For this review, take the finished solid that the model builds, in its own axes (mm). Round coordinates to 2 decimals unless told otherwise and drop trailing zeros.
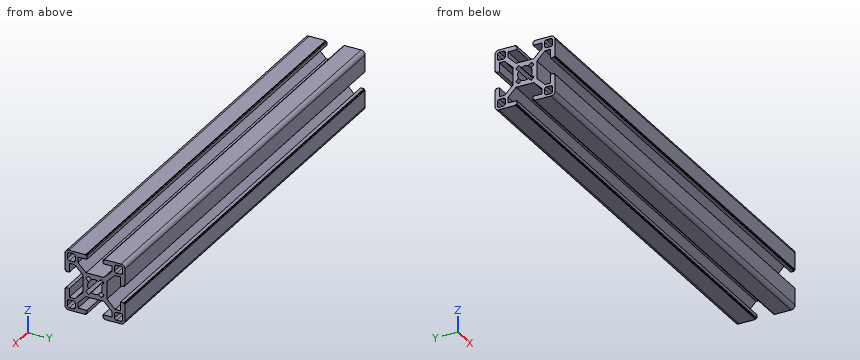
from build123d import *

# Parameters (mm, degrees)
AUFSATZ_LINEAR_AUSTRAGEN1_DEPTH = 220


with BuildPart() as part:
    # Skizze1 → Aufsatz-Linear austragen1 (new body)
    with BuildSketch(Plane(origin=(0, 0, 0), x_dir=(0, 0, -1), z_dir=(1, 0, 0))):
        with BuildLine():
            Line((10.055634919, 8.5), (12.8, 8.5))
            Line((12.8, 8.5), (12.8, 4.05))
            Line((12.8, 4.05), (14.5, 4.05))
            Line((14.5, 4.05), (14.5, 4.651637069))
            Line((14.5, 4.651637069), (15, 4.651637069))
            Line((15, 4.651637069), (15, 13))
            ThreePointArc((15, 13), (14.414213562, 14.414213562), (13, 15))
            Line((13, 15), (4.651637069, 15))
            Line((4.651637069, 15), (4.651637069, 14.5))
            Line((4.651637069, 14.5), (4.05, 14.5))
            Line((4.05, 14.5), (4.05, 12.8))
            Line((4.05, 12.8), (8.5, 12.8))
            Line((8.5, 12.8), (8.5, 10.055634919))
            Line((8.5, 10.055634919), (4.444365081, 6))
            Line((4.444365081, 6), (-4.444365081, 6))
            Line((-4.444365081, 6), (-8.5, 10.055634919))
            Line((-8.5, 10.055634919), (-8.5, 12.8))
            Line((-8.5, 12.8), (-4.05, 12.8))
            Line((-4.05, 12.8), (-4.05, 14.5))
            Line((-4.05, 14.5), (-4.651637069, 14.5))
            Line((-4.651637069, 14.5), (-4.651637069, 15))
            Line((-4.651637069, 15), (-13, 15))
            ThreePointArc((-13, 15), (-14.414213562, 14.414213562), (-15, 13))
            Line((-15, 13), (-15, 4.651637069))
            Line((-15, 4.651637069), (-14.5, 4.651637069))
            Line((-14.5, 4.651637069), (-14.5, 4.05))
            Line((-14.5, 4.05), (-12.8, 4.05))
            Line((-12.8, 4.05), (-12.8, 8.5))
            Line((-12.8, 8.5), (-10.055634919, 8.5))
            Line((-10.055634919, 8.5), (-6, 4.444365081))
            Line((-6, 4.444365081), (-6, -4.444365081))
            Line((-6, -4.444365081), (-10.055634919, -8.5))
            Line((-10.055634919, -8.5), (-12.8, -8.5))
            Line((-12.8, -8.5), (-12.8, -4.05))
            Line((-12.8, -4.05), (-14.5, -4.05))
            Line((-14.5, -4.05), (-14.5, -4.651637069))
            Line((-14.5, -4.651637069), (-15, -4.651637069))
            Line((-15, -4.651637069), (-15, -13))
            ThreePointArc((-15, -13), (-14.414213562, -14.414213562), (-13, -15))
            Line((-13, -15), (-4.651637069, -15))
            Line((-4.651637069, -15), (-4.651637069, -14.5))
            Line((-4.651637069, -14.5), (-4.05, -14.5))
            Line((-4.05, -14.5), (-4.05, -12.8))
            Line((-4.05, -12.8), (-8.5, -12.8))
            Line((-8.5, -12.8), (-8.5, -10.055634919))
            Line((-8.5, -10.055634919), (-4.444365081, -6))
            Line((-4.444365081, -6), (4.444365081, -6))
            Line((4.444365081, -6), (8.5, -10.055634919))
            Line((8.5, -10.055634919), (8.5, -12.8))
            Line((8.5, -12.8), (4.05, -12.8))
            Line((4.05, -12.8), (4.05, -14.5))
            Line((4.05, -14.5), (4.651637069, -14.5))
            Line((4.651637069, -14.5), (4.651637069, -15))
            Line((4.651637069, -15), (13, -15))
            ThreePointArc((13, -15), (14.414213562, -14.414213562), (15, -13))
            Line((15, -13), (15, -4.651637069))
            Line((15, -4.651637069), (14.5, -4.651637069))
            Line((14.5, -4.651637069), (14.5, -4.05))
            Line((14.5, -4.05), (12.8, -4.05))
            Line((12.8, -4.05), (12.8, -8.5))
            Line((12.8, -8.5), (10.055634919, -8.5))
            Line((10.055634919, -8.5), (6, -4.444365081))
            Line((6, -4.444365081), (6, 4.444365081))
            Line((6, 4.444365081), (10.055634919, 8.5))
        make_face()
        with BuildLine():
            ThreePointArc((12.8, 13.8), (13.507106781, 13.507106781), (13.8, 12.8))
            Line((13.8, 12.8), (13.8, 10.8))
            ThreePointArc((13.8, 10.8), (13.507106781, 10.092893219), (12.8, 9.8))
            Line((12.8, 9.8), (10.8, 9.8))
            ThreePointArc((10.8, 9.8), (10.092893219, 10.092893219), (9.8, 10.8))
            Line((9.8, 10.8), (9.8, 12.8))
            ThreePointArc((9.8, 12.8), (10.092893219, 13.507106781), (10.8, 13.8))
            Line((10.8, 13.8), (12.8, 13.8))
        make_face(mode=Mode.SUBTRACT)
        with BuildLine():
            Line((-3.117157854, 4.531371416), (-1.775079755, 3.189293317))
            ThreePointArc((-1.775079755, 3.189293317), (0, 3.65), (1.775079755, 3.189293317))
            Line((1.775079755, 3.189293317), (3.117157854, 4.531371416))
            ThreePointArc((3.117157854, 4.531371416), (3.889087297, 3.889087297), (4.531371416, 3.117157854))
            Line((4.531371416, 3.117157854), (3.189293317, 1.775079755))
            ThreePointArc((3.189293317, 1.775079755), (3.65, 0), (3.189293317, -1.775079755))
            Line((3.189293317, -1.775079755), (4.531371416, -3.117157854))
            ThreePointArc((4.531371416, -3.117157854), (3.889087297, -3.889087297), (3.117157854, -4.531371416))
            Line((3.117157854, -4.531371416), (1.775079755, -3.189293317))
            ThreePointArc((1.775079755, -3.189293317), (0, -3.65), (-1.775079755, -3.189293317))
            Line((-1.775079755, -3.189293317), (-3.117157854, -4.531371416))
            ThreePointArc((-3.117157854, -4.531371416), (-3.889087297, -3.889087297), (-4.531371416, -3.117157854))
            Line((-4.531371416, -3.117157854), (-3.189293317, -1.775079755))
            ThreePointArc((-3.189293317, -1.775079755), (-3.65, 0), (-3.189293317, 1.775079755))
            Line((-3.189293317, 1.775079755), (-4.531371416, 3.117157854))
            ThreePointArc((-4.531371416, 3.117157854), (-3.889087297, 3.889087297), (-3.117157854, 4.531371416))
        make_face(mode=Mode.SUBTRACT)
        with BuildLine():
            ThreePointArc((-13.8, 12.8), (-13.507106781, 13.507106781), (-12.8, 13.8))
            Line((-12.8, 13.8), (-10.8, 13.8))
            ThreePointArc((-10.8, 13.8), (-10.092893219, 13.507106781), (-9.8, 12.8))
            Line((-9.8, 12.8), (-9.8, 10.8))
            ThreePointArc((-9.8, 10.8), (-10.092893219, 10.092893219), (-10.8, 9.8))
            Line((-10.8, 9.8), (-12.8, 9.8))
            ThreePointArc((-12.8, 9.8), (-13.507106781, 10.092893219), (-13.8, 10.8))
            Line((-13.8, 10.8), (-13.8, 12.8))
        make_face(mode=Mode.SUBTRACT)
        with BuildLine():
            ThreePointArc((9.8, -10.8), (10.092893219, -10.092893219), (10.8, -9.8))
            Line((10.8, -9.8), (12.8, -9.8))
            ThreePointArc((12.8, -9.8), (13.507106781, -10.092893219), (13.8, -10.8))
            Line((13.8, -10.8), (13.8, -12.8))
            ThreePointArc((13.8, -12.8), (13.507106781, -13.507106781), (12.8, -13.8))
            Line((12.8, -13.8), (10.8, -13.8))
            ThreePointArc((10.8, -13.8), (10.092893219, -13.507106781), (9.8, -12.8))
            Line((9.8, -12.8), (9.8, -10.8))
        make_face(mode=Mode.SUBTRACT)
        with BuildLine():
            Line((-9.8, -10.8), (-9.8, -12.8))
            ThreePointArc((-9.8, -12.8), (-10.092893219, -13.507106781), (-10.8, -13.8))
            Line((-10.8, -13.8), (-12.8, -13.8))
            ThreePointArc((-12.8, -13.8), (-13.507106781, -13.507106781), (-13.8, -12.8))
            Line((-13.8, -12.8), (-13.8, -10.8))
            ThreePointArc((-13.8, -10.8), (-13.507106781, -10.092893219), (-12.8, -9.8))
            Line((-12.8, -9.8), (-10.8, -9.8))
            ThreePointArc((-10.8, -9.8), (-10.092893219, -10.092893219), (-9.8, -10.8))
        make_face(mode=Mode.SUBTRACT)
    extrude(amount=AUFSATZ_LINEAR_AUSTRAGEN1_DEPTH)


solid = part.part
(1) We need section A-A, the plane x = 26. State how many separate pieces and enclosed holes the cut face has, and give its area (3 significant figures).
Geometry check:
separate pieces: 1
enclosed holes: 5
area: 309 mm2
(2) For line 1 along Y through (x, z) = (66.5, 11.75); line 2 along Z through (x, y) = (149, 13); line 3 along Z through (x, y) = (116.5, 3.75), list the stretches that pass through material, from the lowest coordinate up.
Geometry check:
line 1: y = -15 to -13.8, -9.8 to -8.5, 8.5 to 9.8, 13.8 to 15
line 2: z = -15 to -13.78, -9.82 to -4.05, 4.05 to 9.82, 13.78 to 15
line 3: z = -6 to -4.02, -2.34 to 2.34, 4.02 to 6
(3) For pin 1 Ø0.5 at (x, z) = (80.5, -13.5) entering from +Y; pin 2 Ø2 at (y, z) = (12, 2) entering from +X, all flat-tipped, find the tip position at first contact; note any pin that passes through.
Geometry check:
pin 1: stops at y = 14.98
pin 2: passes through
